Could you check a few things on this model? Use its own coordinates, in mm. Face numbers are marked on the shaded views. A direction names the side the tool comes from. Give positions to 0.01 mm unless a question says otherwise; leave off trailing zeros. Use a Markdown table: item, result. Add a question column.
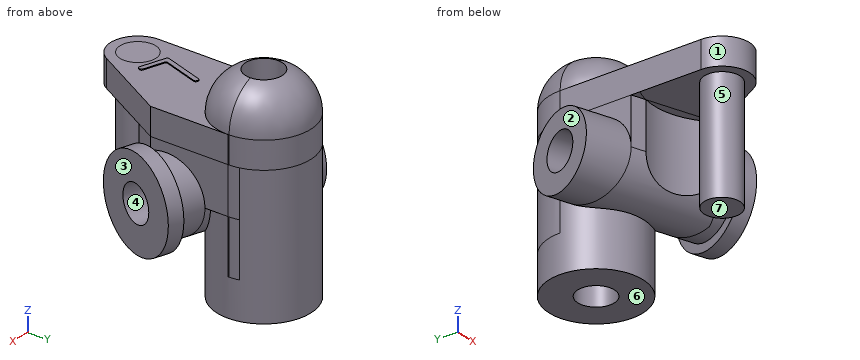
```python
from build123d import *
from build123d.topology import SkipClean

# Parameters (mm, degrees)
BOSS_EXTRU_1_DEPTH       = 1.45
ESQUISSE2_R              = 2.5
BOSS_EXTRU_2_DEPTH       = 2.2
BOSS_EXTRU_3_START       = 7.4
ESQUISSE4_R              = 2.5
BOSS_EXTRU_3_DEPTH       = 11.05
BOSS_EXTRU_4_START       = -1.45
ESQUISSE5_R              = 0.95
BOSS_EXTRU_4_DEPTH       = 7.5
CONG_2_R                 = 2.2
BOSS_EXTRU_5_DEPTH       = 1
BOSS_EXTRU_5_DEPTH_BACK  = 7.45
ENL_V_START              = -5.4
ENL_V_MAT_EXTRU_7_DEPTH  = 5.4
BOSS_EXTRU_14_DEPTH      = 1
BOSS_EXTRU_14_DEPTH_BACK = 7.45
ESQUISSE14_R             = 2
ESQUISSE15_R             = 2.45
BOSS_EXTRU_15_DEPTH      = 0.8
ENL_V_START_2            = -6.05
ESQUISSE16_R             = 3.6
ESQUISSE16_R_2           = 0.95
ENL_V_MAT_EXTRU_9_DEPTH  = 6.05
ESQUISSE17_R             = 0.975
ENL_V_MAT_EXTRU_10_DEPTH = 12.8
ESQUISSE18_R             = 0.975
ENL_V_MAT_EXTRU_11_DEPTH = 12.8
BOSS_EXTRU_16_DEPTH      = 0.05
SCALE1_SCALE             = 6.5


with BuildPart() as part:
    # Esquisse1 → Boss.-Extru.1 (new body)
    with BuildSketch(Plane.XY):
        with BuildLine():
            Line((-2.499269345, 0.060437906), (-2.682459021, -7.514946015))
            ThreePointArc((-2.682459021, -7.514946015), (-1.629243216, -8.944775402), (0.018499188, -8.282491037))
            Line((0.018499188, -8.282491037), (2.398777572, -4.216041966))
            Line((2.398777572, -4.216041966), (2.499269345, -0.060437906))
            ThreePointArc((2.499269345, -0.060437906), (0.060437906, 2.499269345), (-2.499269345, 0.060437906))
        make_face()
    extrude(amount=BOSS_EXTRU_1_DEPTH)

    # Esquisse2 → Boss.-Extru.2 (add)
    with BuildSketch(Plane.XY.offset(1.45)):
        with Locations(Location((0, 0, 0), (0, 0, 178.614730271))):
            Circle(ESQUISSE2_R)
    extrude(amount=BOSS_EXTRU_2_DEPTH)

    # Esquisse4 → Boss.-Extru.3 (add)
    with SkipClean():  # the faces are left unmerged after this step: merging them gives an invalid solid
        with BuildSketch(Plane(origin=(0, 0, 0), x_dir=(-1, 0, 0), z_dir=(0, 0, -1)).offset(BOSS_EXTRU_3_START)):
            with Locations(Location((0, 0, 0), (0, 0, 180))):
                Circle(ESQUISSE4_R)
        extrude(amount=-BOSS_EXTRU_3_DEPTH)
    add(part.part.scale(1), mode=Mode.REPLACE)  # the faces are merged on a copy

    # Esquisse5 → Boss.-Extru.4 (add)
    with SkipClean():  # the faces are left unmerged after this step: merging them gives an invalid solid
        with BuildSketch(Plane(origin=(0, 0, 0), x_dir=(-1, 0, 0), z_dir=(0, 0, -1)).offset(BOSS_EXTRU_4_START)):
            with Locations(Location((1.232882801, -7.55, 0), (0, 0, 180))):
                Circle(ESQUISSE5_R)
        extrude(amount=BOSS_EXTRU_4_DEPTH)

    # Congé2
    cong_2_edges = [part.edges().sort_by_distance(p)[0] for p in [
        (0.030221161, 2.49981733, 3.65),
    ]]
    fillet(cong_2_edges, radius=CONG_2_R - 0.0001)  # a hair under: the kernel refuses the full size

    # Esquisse6 → Boss.-Extru.5 (add, two sides: drawn at the far end of the back side and taken through both)
    with BuildSketch(Plane(origin=(-2.358270057, 0.829796565, 0), x_dir=(0, 0, 1), z_dir=(-0.9433080226536918, 0.3319186261678939, 0)).offset(-BOSS_EXTRU_5_DEPTH_BACK)):
        with BuildLine():
            Line((-2.5, -4.4), (0, -4.4))
            Line((0, -4.4), (0, 1.297884729))
            Line((0, 1.297884729), (-2.5, 1.297884729))
            Line((-2.5, 1.297884729), (-2.5, -0.4))
            ThreePointArc((-2.5, -0.4), (-4.5, -2.4), (-2.5, -4.4))
        make_face()
    extrude(amount=BOSS_EXTRU_5_DEPTH + BOSS_EXTRU_5_DEPTH_BACK)

    # Esquisse13 → Enlèv. mat.-Extru.7 (cut)
    with SkipClean():  # the faces are left unmerged after this step: merging them gives an invalid solid
        with BuildSketch(Plane.XY.offset(ENL_V_START)):
            with BuildLine():
                Line((-1.584775977, 1.933516253), (-2.870785963, 2.386020269))
                Line((-2.870785963, 2.386020269), (-4.762020034, -2.988840108))
                Line((-4.762020034, -2.988840108), (-2.591476667, -3.752581914))
                Line((-2.591476667, -3.752581914), (-2.499269345, 0.060437906))
                ThreePointArc((-2.499269345, 0.060437906), (-2.246544496, 1.096830811), (-1.584775977, 1.933516253))
            make_face()
            with BuildLine():
                Line((1.771456427, -5.28775253), (3.208932757, -5.793552499))
                Line((3.208932757, -5.793552499), (5.100166828, -0.418692123))
                Line((5.100166828, -0.418692123), (2.446360209, 0.515093901))
                ThreePointArc((2.446360209, 0.515093901), (2.489502388, 0.228862104), (2.499269345, -0.060437906))
                Line((2.499269345, -0.060437906), (2.398777572, -4.216041966))
                Line((2.398777572, -4.216041966), (1.771456427, -5.28775253))
            make_face()
        extrude(amount=ENL_V_MAT_EXTRU_7_DEPTH, mode=Mode.SUBTRACT)

    # Esquisse14 → Boss.-Extru.14 (add, two sides: drawn at the far end of the back side and taken through both)
    with BuildSketch(Plane(origin=(-2.358270057, 0.829796565, 0), x_dir=(0, 0, 1), z_dir=(-0.9433080226536918, 0.3319186261678939, 0)).offset(-BOSS_EXTRU_14_DEPTH_BACK)):
        with Locations(Location((-2.5, -2.4, 0), (0, 0, 270))):
            Circle(ESQUISSE14_R)
    extrude(amount=BOSS_EXTRU_14_DEPTH + BOSS_EXTRU_14_DEPTH_BACK)

    # Esquisse15 → Boss.-Extru.15 (add)
    with BuildSketch(Plane(origin=(4.669374712, -1.6429972, 0), x_dir=(0, 0, -1), z_dir=(0.9433080226536918, -0.33191862616789397, 0))):
        with Locations(Location((2.5, -2.4, 0), (0, 0, 90))):
            Circle(ESQUISSE15_R)
    extrude(amount=-BOSS_EXTRU_15_DEPTH)

    # Esquisse16 → Enlèv. mat.-Extru.9 (cut)
    with BuildSketch(Plane(origin=(0, 0, -6.05), x_dir=(-1, 0, 0), z_dir=(0, 0, -1)).offset(ENL_V_START_2)):
        with Locations((1.232882801, -7.55)):
            Circle(ESQUISSE16_R)
        with Locations(Location((1.232882801, -7.55, 0), (0, 0, 180))):
            Circle(ESQUISSE16_R_2, mode=Mode.SUBTRACT)
    extrude(amount=ENL_V_MAT_EXTRU_9_DEPTH, mode=Mode.SUBTRACT)

    # Esquisse17 → Enlèv. mat.-Extru.10 (cut)
    with BuildSketch(Plane(origin=(0, 0, -7.4), x_dir=(-1, 0, 0), z_dir=(0, 0, -1))):
        Circle(ESQUISSE17_R)
    extrude(amount=-ENL_V_MAT_EXTRU_10_DEPTH, mode=Mode.SUBTRACT)

    # Esquisse18 → Enlèv. mat.-Extru.11 (cut)
    with BuildSketch(Plane(origin=(4.669374712, -1.6429972, 0), x_dir=(0, 0, -1), z_dir=(0.9433080226536918, -0.33191862616789397, 0))):
        with Locations(Location((2.5, -2.4, 0), (0, 0, 90))):
            Circle(ESQUISSE18_R)
    extrude(amount=-ENL_V_MAT_EXTRU_11_DEPTH, mode=Mode.SUBTRACT)

    # Esquisse19 → Boss.-Extru.16 (add)
    with BuildSketch(Plane.XY.offset(1.45)):
        with BuildLine():
            Line((-0.741145926, -3.994756307), (-1.473216513, -6.075290521))
            ThreePointArc((-1.473216513, -6.075290521), (-1.469057852, -6.151714142), (-1.412077574, -6.202813186))
            Line((-1.412077574, -6.202813186), (-0.127522665, -6.654805208))
            ThreePointArc((-0.127522665, -6.654805208), (-0.051099043, -6.650646547), (0, -6.593666268))
            Line((0, -6.593666268), (0.016595931, -6.546500867))
            ThreePointArc((0.016595931, -6.546500867), (0.01243727, -6.470077246), (-0.044543008, -6.418978202))
            Line((-0.044543008, -6.418978202), (-1.093270911, -6.049965837))
            ThreePointArc((-1.093270911, -6.049965837), (-1.15025119, -5.998866793), (-1.154409851, -5.922443172))
            Line((-1.154409851, -5.922443172), (-0.50531892, -4.077735963))
            ThreePointArc((-0.50531892, -4.077735963), (-0.509477582, -4.001312342), (-0.56645786, -3.950213298))
            Line((-0.56645786, -3.950213298), (-0.613623261, -3.933617367))
            ThreePointArc((-0.613623261, -3.933617367), (-0.690046883, -3.937776028), (-0.741145926, -3.994756307))
        make_face()
    extrude(amount=BOSS_EXTRU_16_DEPTH)


with BuildPart() as part_1:
    # Scale1: scaled about (-0.062378665, -1.819814111, -1.884608328)
    add(part.part.scale(SCALE1_SCALE).moved(Location((0.343082657, 10.00897761, 10.365345804))))


solid = part_1.part
```
1) We'd pull the mould along X, two halves only. Please class the marked faces 1, 2, 3 and 4: pulls with the +X half, pulls with the -X half, needs draft (parallel to the pull), parting line crosses it, or undercut.
2) Suppose I cut it at A-A on z = -3. Count the separate pieces of the cut face and the enclosed holes in it, and give its area (3 significant figures).
3) Please list where these lines run through material, in increasing order: line 1 (Y direction, x = 3, z = -0.5); line 2 (X direction, y = 9.5, z = 18); line 3 (Z direction, x = -11, y = -2.5). Write a range as from..to.
4) For pin 1 (2.5 mm diameter, centred on x = -13, y = -15.5, fed in from -Z); pin 2 (10 mm diameter, centred on x = -10, y = -36.5, fed in from +Z); pin 3 (2.5 mm diameter, centred on x = 0, y = -20, fed in from -Z); pin 4 (12 mm diameter, centred on x = -23, y = -33.5, fed in from +Z), each with a flat end and sliding along its axis, tell me the tip position at first contact or that it passes through.
5) For the marked faces 5, 6 and 7, which set-ups out of +Z, -Z, +X, -X, +Y, -Y let a thin tool reach every point of the face, with its end or its side?
Values found:
| question | item | result |
|---|---|---|
| 1 | face 1 | parting line crosses it |
| 1 | face 2 | pulls with the -X half |
| 1 | face 3 | pulls with the +X half |
| 1 | face 4 | undercut |
| 2 | separate pieces | 3 |
| 2 | enclosed holes | 1 |
| 2 | area | 1,270 mm^2 |
| 3 | line 1 | y = -18.24..-11.01, -3.92..4.26, 15.76..26.04 |
| 3 | line 2 | x = -15.92..-5.97, 6.66..16.59 |
| 3 | line 3 | z = -18.88..-12.22, 0.45..19.79 |
| 4 | pin 1 | stops at z = -11.67 |
| 4 | pin 2 | stops at z = 19.79 |
| 4 | pin 3 | stops at z = 10.37 |
| 4 | pin 4 | passes through |
| 5 | face 5 | -Z |
| 5 | face 6 | -Z, +X, -X, +Y, -Y |
| 5 | face 7 | -Z, +X, -X, -Y |
